Check sheet for the modelled part. Datum: model origin and axes. Units: mm. A direction names the side the tool comes from. Round coordinates to 2 decimals unless told otherwise and drop trailing zeros. Write each loop counter-clockwise with the first axis right and the second up, starting at its lowest first coordinate (ties: lowest second). Pieces come first, ordered by that corner, then holes. Notation, with made-up numbers: (-21.5, 81) - (34.5, 81) arc R10 ccw to (34.5, 87) - close; hole circle Ø1 at (-29, 56). An arc over 180 degrees is marked (long way). Answer as a JSON object with one key per item and string values. Group by question number.
Item 1: Sectioned sample at A-A on y = 20. Record the boundary of the cut face in (x, z), plus the area to 3 significant figures.
Item 2: Set-up check for faces 1 (the flat face through (8, 10, 12)), 2 (the flat face through (15.5, 25, 12)), 3 (the flat face through (0, 25, 12)): record each of +Z, -Z, +X, -X, +Y, -Y from which the full face is reachable in a straight line by a thin tool's end or side.
Item 3: Gauge pin test, flat ends, axial feed: P1, Ø10, axis at y = 23, z = 11.5, coming from the +X side; P2, Ø6, axis at y = 32.5, z = 17.5, coming from the +X side; P3, Ø16, axis at y = 27, z = 8.5, coming from the -X side. Record the tip position at first contact, or that the pin passes through.
Item 4: Release check for a two-part mould opening along Z. For faces 4 (the flat face through (8, 40, 49)), 5 (the flat face through (8, 20, 90)), 6 (the cylindrical face through (7.642, 15.564, 12.307)) record: pulls with the +Z half, pulls with the -Z half, needs draft (parallel to the pull), parting line crosses it, or undercut.
Item 5: Sectioned sample at C-C on y = 5. Record the boundary of the cut face in (x, z).
Item 6: Thickness scan on line 1 (Y direction, x = 3, z = 10); line 2 (X direction, y = 19, z = 18.5); line 3 (Z direction, x = 24, y = 11). Record the ranges inside material, lowest first.
Item 7: Sectioned sample at D-D on y = 36. Record the boundary of the cut face in (x, z).
Item 8: Sectioned sample at B-B on x = 1.5. Record the boundary of the cut face in (y, z).
```python
from build123d import *

# Parameters (mm, degrees)
BOSS_EXTRUDE2_DEPTH = 40
FILLET1_R           = 10
FILLET2_R           = 10
FILLET3_R           = 10
SKETCH3_W           = 20
SKETCH3_H           = 10
CUT_EXTRUDE2_DEPTH  = 40
FILLET4_R           = 5
FILLET5_R           = 5
FILLET6_R           = 5
SKETCH2_R           = 5
CUT_EXTRUDE3_DEPTH  = 28


with BuildPart() as part:
    # Sketch1 → Boss-Extrude2 (new body)
    with BuildSketch(Plane(origin=(0, 0, 0), x_dir=(1, 0, 0), z_dir=(0, 1, 0))):
        Polygon((0, 0), (15.5, 0), (15.5, -20), (40.75, -20), (40.75, -90), (-25.25, -90), (-25.25, -20), (0, -20), align=None)
    extrude(amount=BOSS_EXTRUDE2_DEPTH)

    # Fillet1
    fillet1_edges = [part.edges().sort_by_distance(p)[0] for p in [
        (7.75, 40, 0),
    ]]
    fillet(fillet1_edges, radius=FILLET1_R)

    # Fillet2
    fillet2_edges = [part.edges().sort_by_distance(p)[0] for p in [
        (40.75, 20, 90),
    ]]
    fillet(fillet2_edges, radius=FILLET2_R)

    # Fillet3
    fillet3_edges = [part.edges().sort_by_distance(p)[0] for p in [
        (-25.25, 20, 90),
    ]]
    fillet(fillet3_edges, radius=FILLET3_R)

    # Sketch3 → Cut-Extrude2 (cut)
    with BuildSketch(Plane.ZY):
        with Locations((10, 5)):
            Rectangle(SKETCH3_W, SKETCH3_H)
    extrude(amount=-CUT_EXTRUDE2_DEPTH, mode=Mode.SUBTRACT)

    # Fillet4
    fillet4_edges = [part.edges().sort_by_distance(p)[0] for p in [
        (7.75, 10, 0),
    ]]
    fillet(fillet4_edges, radius=FILLET4_R)

    # Fillet5
    fillet5_edges = [part.edges().sort_by_distance(p)[0] for p in [
        (-25.25, 20, 20),
    ]]
    fillet(fillet5_edges, radius=FILLET5_R)

    # Fillet6
    fillet6_edges = [part.edges().sort_by_distance(p)[0] for p in [
        (40.75, 20, 20),
    ]]
    fillet(fillet6_edges, radius=FILLET6_R)

    # Sketch2 → Cut-Extrude3 (cut)
    with BuildSketch(Plane.ZY):
        with Locations((10, 20)):
            Circle(SKETCH2_R)
    extrude(amount=-CUT_EXTRUDE3_DEPTH, mode=Mode.SUBTRACT)


solid = part.part
```
Completed:
{
 "1": {"outline": "(-25.25, 25) arc R5 ccw to (-20.25, 20) - (0, 20) - (0, 15) - (15.5, 15) - (15.5, 20) - (35.75, 20) arc R5 ccw to (40.75, 25) - (40.75, 80) arc R10 ccw to (30.75, 90) - (-15.25, 90) arc R10 ccw to (-25.25, 80) - close; (0, 0) - (15.5, 0) - (15.5, 5) - (0, 5) - close", "area": "4,720 mm²"},
 "2": {"face 1": "-Z, +X, -X, -Y", "face 2": "-Z, +X, +Y, -Y", "face 3": "-Z, -X, +Y, -Y"},
 "3": {"P1": "x = 15.5", "P2": "x = 37.93", "P3": "x = 0"},
 "4": {"face 4": "needs draft", "face 5": "pulls with the +Z half", "face 6": "undercut"},
 "5": {"outline": "(-25.25, 25) arc R5 ccw to (-20.25, 20) - (35.75, 20) arc R5 ccw to (40.75, 25) - (40.75, 80) arc R10 ccw to (30.75, 90) - (-15.25, 90) arc R10 ccw to (-25.25, 80) - close"},
 "6": {"line 1": "10 to 15, 25 to 40", "line 2": "0 to 15.5", "line 3": "20 to 90"},
 "7": {"outline": "(-25.25, 25) arc R5 ccw to (-20.25, 20) - (0, 20) - (0, 2) - (15.5, 2) - (15.5, 20) - (35.75, 20) arc R5 ccw to (40.75, 25) - (40.75, 80) arc R10 ccw to (30.75, 90) - (-15.25, 90) arc R10 ccw to (-25.25, 80) - close"},
 "8": {"outline": "(0, 20) - (10, 20) - (10, 5) arc R5 ccw to (15, 0) - (30, 0) arc R10 ccw to (40, 10) - (40, 90) - (0, 90) - close; hole circle Ø10 at (20, 10)"}
}
